Check sheet for the modelled part. Datum: model origin and axes. Units: mm. Face numbers are marked on the shaded views. A direction names the side the tool comes from. Round coordinates to 2 decimals unless told otherwise and drop trailing zeros. Write each loop counter-clockwise with the first axis right and the second up, starting at its lowest first coordinate (ties: lowest second). Pieces come first, ordered by that corner, then holes. Notation, with made-up numbers: (36, 30) -> (46, 30) arc R20 cw to (46, 56) -> close; hole circle Ø1 at (42.5, -25.5). An arc over 180 degrees is marked (long way). Write item = value, one per line.
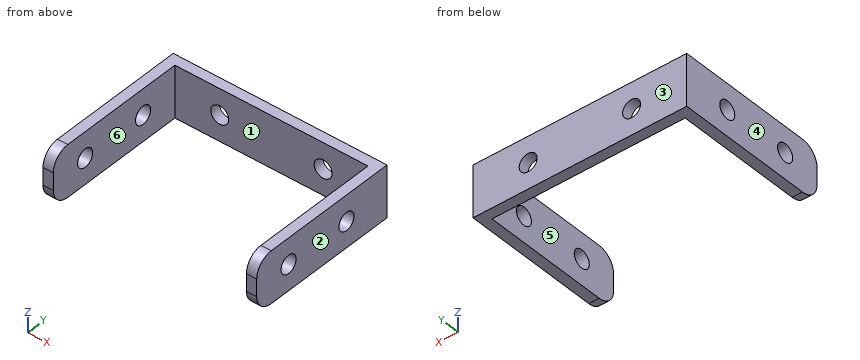
from build123d import *

# Parameters (mm, degrees)
RESSALTO_EXTRUS_O1_DEPTH = 15
ESBO_O2_R                = 2.6
CORTE_EXTRUS_O1_DEPTH    = 15
ESBO_O3_R                = 2.6
CORTE_EXTRUS_O2_DEPTH    = 63
FILETE1_R                = 5


with BuildPart() as part:
    # Esboço1 → Ressalto-extrusão1 (new body)
    with BuildSketch(Plane.XY):
        Polygon((-31, 0), (-28, 0), (-28, 42), (28, 42), (28, 0), (31, 0), (31, 45), (-31, 45), align=None)
    extrude(amount=RESSALTO_EXTRUS_O1_DEPTH)

    # Esboço2 → Corte-extrusão1 (cut)
    with BuildSketch(Plane(origin=(0, 45, 0), x_dir=(1, 0, 0), z_dir=(0, 1, 0))):
        with Locations((-15, -7.5)):
            Circle(ESBO_O2_R)
        with Locations((15, -7.5)):
            Circle(ESBO_O2_R)
    extrude(amount=-CORTE_EXTRUS_O1_DEPTH, mode=Mode.SUBTRACT)

    # Esboço3 → Corte-extrusão2 (cut, through all)
    with BuildSketch(Plane(origin=(31, 0, 0), x_dir=(0, 0, -1), z_dir=(1, 0, 0))):
        with Locations((-7.5, 11)):
            Circle(ESBO_O3_R)
        with Locations((-7.5, 31)):
            Circle(ESBO_O3_R)
    extrude(amount=-CORTE_EXTRUS_O2_DEPTH, mode=Mode.SUBTRACT)

    # Filete1
    filete1_edges = [part.edges().sort_by_distance(p)[0] for p in [
        (-29.5, 0, 0),
        (29.5, 0, 15),
        (-29.5, 0, 15),
        (29.5, 0, 0),
    ]]
    fillet(filete1_edges, radius=FILETE1_R)


solid = part.part
(1) Sectioned sample at B-B on z = 7.5. Count the separate pieces of the cut face and the enclosed holes in it, then the cut area to 3 significant figures.
Worked answers:
separate_pieces = 7
enclosed_holes = 0
area = 344 mm²
(2) Access from +Z, -Z, +X, -X, +Y, -Y to the whole of each face (thin tool, end or side, straight path). Record for the marked faces 1 and 2.
Worked answers:
face_1 = +Z, -Z, -Y
face_2 = +Z, -Z, +X, +Y, -Y
(3) Release check for a two-part mould opening along X. For the marked faces 3, 4, 5 and 6 record: pulls with the +X half, pulls with the -X half, needs draft (parallel to the pull), parting line crosses it, or undercut.
Worked answers:
face_3 = needs draft
face_4 = pulls with the -X half
face_5 = undercut
face_6 = undercut
(4) Material ranges on L1, parallel to Y at x = -29.4, z = 7.5; L2, parallel to X at y = 43.9, z = 7.5; L3, parallel to Z at x = 15, y = 44, recorded low to high. Write a range as [from, to].
Worked answers:
L1 = [0, 8.4], [13.6, 28.4], [33.6, 45]
L2 = [-31, -17.6], [-12.4, 12.4], [17.6, 31]
L3 = [0, 4.9], [10.1, 15]
(5) Go/stop test with flat-tipped pins: P1, Ø4.5, axis at x = -15, z = 7.5, coming from the -Y side; P2, Ø7, axis at y = 31, z = 7.5, coming from the +X side; P3, Ø3, axis at x = 23, z = 9, coming from the -Y side. Record where each tip stops, or that it passes through.
Worked answers:
P1 = through
P2 = 31
P3 = 42
(6) Sectioned sample at A-A on x = 15. Enter the section's corners in (y, z), then the cut area to 3 significant figures.
Worked answers:
outline = (42, 0) -> (45, 0) -> (45, 4.9) -> (42, 4.9) -> close; (42, 10.1) -> (45, 10.1) -> (45, 15) -> (42, 15) -> close
area = 29.4 mm²
(7) Sectioned sample at D-D on y = 31. Enter the section's corners in (x, z), then the cut area to 3 significant figures.
Worked answers:
outline = (-31, 0) -> (-28, 0) -> (-28, 4.9) -> (-31, 4.9) -> close; (-31, 10.1) -> (-28, 10.1) -> (-28, 15) -> (-31, 15) -> close; (28, 0) -> (31, 0) -> (31, 4.9) -> (28, 4.9) -> close; (28, 10.1) -> (31, 10.1) -> (31, 15) -> (28, 15) -> close
area = 58.8 mm²
(8) Sectioned sample at C-C on y = 39. Enter the section's corners in (x, z), then the cut area to 3 significant figures.
Worked answers:
outline = (-31, 0) -> (-28, 0) -> (-28, 15) -> (-31, 15) -> close; (28, 0) -> (31, 0) -> (31, 15) -> (28, 15) -> close
area = 90.0 mm²
